The listing builds one solid part. Answer for the finished solid, in the listing's coordinates (mm). A direction names the side the tool comes from. Round coordinates to 2 decimals unless told otherwise and drop trailing zeros. Write each loop counter-clockwise with the first axis right and the second up, starting at its lowest first coordinate (ties: lowest second). Pieces come first, ordered by that corner, then holes. Notation, with made-up numbers: (61.25, 67) - (68.25, 67) arc R18 cw to (68.25, 81) - close; hole circle Ø5 at (-35.5, 46). An arc over 180 degrees is marked (long way). Answer in a Markdown table with one row per item.
from build123d import *

# Parameters (mm, degrees)
BOSS_EXTRUDE1_DEPTH = 25
BOSS_EXTRUDE2_START = 12
SKETCH1_3_R         = 4.5
BOSS_EXTRUDE2_DEPTH = 12
CUT_EXTRUDE1_REACH  = 131.64
CUT_EXTRUDE2_REACH  = 199.844
SKETCH3_R           = 3.5


with BuildPart() as part:
    # Sketch1 → Boss-Extrude1 (new, symmetric)
    with BuildSketch(Plane.XY):
        with BuildLine():
            Line((18.5, 11), (18.5, 42))
            ThreePointArc((18.5, 42), (0, 60.5), (-18.5, 42))
            Line((-18.5, 42), (-18.5, 11))
            Line((-18.5, 11), (-57, 11))
            Line((-57, 11), (-57, 27))
            Line((-57, 27), (-62, 27))
            Line((-62, 27), (-62, 43))
            Line((-62, 43), (-72, 43))
            Line((-72, 43), (-72, 0))
            Line((-72, 0), (108, 0))
            Line((108, 0), (108, 11))
            Line((108, 11), (18.5, 11))
        make_face()
        with BuildLine():
            ThreePointArc((2.5, 31.287857357), (0, 53), (-2.5, 31.287857357))
            Line((-2.5, 31.287857357), (-2.5, 25.287857357))
            Line((-2.5, 25.287857357), (2.5, 25.287857357))
            Line((2.5, 25.287857357), (2.5, 31.287857357))
        make_face(mode=Mode.SUBTRACT)
    extrude(amount=BOSS_EXTRUDE1_DEPTH, both=True)

    # Sketch1_3 → Boss-Extrude2 (add)
    with BuildSketch(Plane.XY.offset(BOSS_EXTRUDE2_START)):
        with BuildLine():
            ThreePointArc((0.735842557, 60.485360038), (10.611164072, 57.154312819), (17.118883443, 49.013831311))
            Line((17.118883443, 49.013831311), (26.545966406, 62.477101054))
            ThreePointArc((26.545966406, 62.477101054), (24.090210327, 76.40438586), (10.16292552, 73.948629781))
            Line((10.16292552, 73.948629781), (0.735842557, 60.485360038))
        make_face()
        with Locations((18.354445963, 68.212865417)):
            Circle(SKETCH1_3_R, mode=Mode.SUBTRACT)
    extrude(amount=-BOSS_EXTRUDE2_DEPTH)

    # Sketch2 → Cut-Extrude1 (cut, up to next)
    with BuildSketch(Plane(origin=(0, 11, 0), x_dir=(1, 0, 0), z_dir=(0, 1, 0)), mode=Mode.PRIVATE) as cut_extrude1_sk1:
        with BuildLine():
            Line((58, -12), (83, -12))
            ThreePointArc((83, -12), (95, 0), (83, 12))
            Line((83, 12), (58, 12))
            ThreePointArc((58, 12), (46, 0), (58, -12))
        make_face()
    cut_extrude1_tool1 = extrude(cut_extrude1_sk1.sketch, amount=-CUT_EXTRUDE1_REACH, mode=Mode.PRIVATE) & part.part
    # Sketch2 → Cut-Extrude1 (cut, up to next)
    with BuildSketch(Plane(origin=(0, 11, 0), x_dir=(1, 0, 0), z_dir=(0, 1, 0)), mode=Mode.PRIVATE) as cut_extrude1_sk2:
        with BuildLine():
            ThreePointArc((83, 25), (100.677669542, 17.677669518), (108, -3.4e-08))
            Line((108, -3.4e-08), (108, 25))
            Line((108, 25), (83, 25))
        make_face()
    cut_extrude1_tool2 = extrude(cut_extrude1_sk2.sketch, amount=-CUT_EXTRUDE1_REACH, mode=Mode.PRIVATE) & part.part
    # Sketch2 → Cut-Extrude1 (cut, up to next)
    with BuildSketch(Plane(origin=(0, 11, 0), x_dir=(1, 0, 0), z_dir=(0, 1, 0)), mode=Mode.PRIVATE) as cut_extrude1_sk3:
        with BuildLine():
            ThreePointArc((108, -3.4e-08), (100.677669518, -17.677669542), (83, -25))
            Line((83, -25), (108, -25))
            Line((108, -25), (108, -3.4e-08))
        make_face()
    cut_extrude1_tool3 = extrude(cut_extrude1_sk3.sketch, amount=-CUT_EXTRUDE1_REACH, mode=Mode.PRIVATE) & part.part
    add(cut_extrude1_tool1.solids().sort_by_distance((70.5, 11, 0))[0], mode=Mode.SUBTRACT)
    add(cut_extrude1_tool2.solids().sort_by_distance((102.415802, 11, -19.415802))[0], mode=Mode.SUBTRACT)
    add(cut_extrude1_tool3.solids().sort_by_distance((102.415802, 11, 19.415802))[0], mode=Mode.SUBTRACT)

    # Sketch3 → Cut-Extrude2 (cut, up to next)
    with BuildSketch(Plane.ZY.offset(72), mode=Mode.PRIVATE) as cut_extrude2_sk1:
        with Locations((15, 33)):
            Circle(SKETCH3_R)
    cut_extrude2_tool1 = extrude(cut_extrude2_sk1.sketch, amount=-CUT_EXTRUDE2_REACH, mode=Mode.PRIVATE) & part.part
    # Sketch3 → Cut-Extrude2 (cut, up to next)
    with BuildSketch(Plane.ZY.offset(72), mode=Mode.PRIVATE) as cut_extrude2_sk2:
        with BuildLine():
            ThreePointArc((15, 43), (22.071067812, 40.071067812), (25, 33))
            Line((25, 33), (25, 43))
            Line((25, 43), (15, 43))
        make_face()
    cut_extrude2_tool2 = extrude(cut_extrude2_sk2.sketch, amount=-CUT_EXTRUDE2_REACH, mode=Mode.PRIVATE) & part.part
    # Sketch3 → Cut-Extrude2 (cut, up to next)
    with BuildSketch(Plane.ZY.offset(72), mode=Mode.PRIVATE) as cut_extrude2_sk3:
        with Locations((-15, 33)):
            Circle(SKETCH3_R)
    cut_extrude2_tool3 = extrude(cut_extrude2_sk3.sketch, amount=-CUT_EXTRUDE2_REACH, mode=Mode.PRIVATE) & part.part
    # Sketch3 → Cut-Extrude2 (cut, up to next)
    with BuildSketch(Plane.ZY.offset(72), mode=Mode.PRIVATE) as cut_extrude2_sk4:
        with BuildLine():
            ThreePointArc((-25, 33), (-22.071067778, 40.071067846), (-14.999999905, 43))
            Line((-14.999999905, 43), (-25, 43))
            Line((-25, 43), (-25, 33))
        make_face()
    cut_extrude2_tool4 = extrude(cut_extrude2_sk4.sketch, amount=-CUT_EXTRUDE2_REACH, mode=Mode.PRIVATE) & part.part
    add(cut_extrude2_tool1.solids().sort_by_distance((-72, 33, 15))[0], mode=Mode.SUBTRACT)
    add(cut_extrude2_tool2.solids().sort_by_distance((-72, 40.766321, 22.766321))[0], mode=Mode.SUBTRACT)
    add(cut_extrude2_tool3.solids().sort_by_distance((-72, 33, -15))[0], mode=Mode.SUBTRACT)
    add(cut_extrude2_tool4.solids().sort_by_distance((-72, 40.766321, -22.766321))[0], mode=Mode.SUBTRACT)


solid = part.part
(1) Section A-A (x = 72) is taken. Give the vertices of the cut face in (y, z).
Checked values:
| item | result |
|---|---|
| outline | (0, -25) - (11, -25) - (11, -12) - (0, -12) - close; (0, 12) - (11, 12) - (11, 25) - (0, 25) - close |
(2) Flat-ended cylindrical pins translate along their axes: pin 1 (2.5 mm diameter, centred on x = -59.5, z = -11, fed in from +Y); pin 2 (14 mm diameter, centred on x = 14.5, y = 67, fed in from +Z); pin 3 (15 mm diameter, centred on x = 47.5, z = 6, fed in from +Y); pin 4 (5.5 mm diameter, centred on x = 18.35, y = 68.21, fed in from +Z). Find the tip coordinate at first contact, or state that the pin passes through.
Checked values:
| item | result |
|---|---|
| pin 1 | stops at y = 27 |
| pin 2 | stops at z = 12 |
| pin 3 | stops at y = 11 |
| pin 4 | passes through |
(3) For a pull along Z with two mould halves and no side action, classify faces 4 (the flat face through (14, 64, 0)), 5 (the flat face through (70, 6, 12)), 6 (the flat face through (-59, 27, 0)) as pulls with the +Z half, pulls with the -Z half, needs draft (parallel to the pull), parting line crosses it, or undercut.
Checked values:
| item | result |
|---|---|
| face 4 | pulls with the -Z half |
| face 5 | undercut |
| face 6 | needs draft |
(4) Section B-B (z = 8) is taken. Give the vertices of the cut face in (x, y), and give its area (3 significant figures).
Checked values:
| item | result |
|---|---|
| outline | (-72, 0) - (49.06, 0) - (49.06, 11) - (18.5, 11) - (18.5, 42) arc R18.5 ccw to (17.12, 49.01) - (26.55, 62.48) arc R10 ccw to (10.16, 73.95) - (0.74, 60.49) arc R18.5 ccw to (-18.5, 42) - (-18.5, 11) - (-57, 11) - (-57, 27) - (-62, 27) - (-62, 43) - (-72, 43) - close; (91.94, 0) - (106.69, 0) - (106.69, 11) - (91.94, 11) - close; hole (-2.5, 25.29) - (2.5, 25.29) - (2.5, 31.29) arc R11 ccw (long way) to (-2.5, 31.29) - close; hole circle Ø9 at (18.35, 68.21) |
| area | 3,550 mm2 |
(5) Section D-D (x = -52) is taken. Give the vertices of the cut face in (y, z).
Checked values:
| item | result |
|---|---|
| outline | (0, -25) - (11, -25) - (11, 25) - (0, 25) - close |
(6) Find the intervals of material crossed by line 1 (X direction, y = 26, z = -1.5); line 2 (Y direction, x = 0, z = -4); line 3 (X direction, y = 41, z = -19), in increasing order.
Checked values:
| item | result |
|---|---|
| line 1 | x = -72 to -57, -18.5 to -2.5, 2.5 to 18.5 |
| line 2 | y = 0 to 25.29, 53 to 60.5 |
| line 3 | x = -72 to -62, -18.5 to -10.95, 10.95 to 18.5 |
(7) For faces 1 (the cylindrical face through (-67.07, 40.15, 21.99)), 2 (the flat face through (-57, 19, 0)), 3 (the flat face through (21.8, 55.7, 6.1)), determine the directions among +Z, -Z, +X, -X, +Y, -Y from which every point of the face is accessible in a straight line to the end or side of a thin tool.
Checked values:
| item | result |
|---|---|
| face 1 | +Z, -X, +Y |
| face 2 | +Z, -Z, +Y |
| face 3 | +Z, -Z, +X |
(8) Section C-C (y = 66) is taken. Give the vertices of the cut face in (x, z).
Checked values:
| item | result |
|---|---|
| outline | (4.6, 0) - (14.44, 0) - (14.44, 12) - (4.6, 12) - close; (22.27, 0) - (28.11, 0) - (28.11, 12) - (22.27, 12) - close |
